The drawing under review shows one solid part. Ordinate dimensions are in mm from its lowest x, y, z. Coordinates: 2 decimals unless noted, no trailing zeros. Loops run counter-clockwise (first coordinate to the right, second up) from the corner with the lowest first, then second, coordinate; pieces in that order, holes last. Notation, with made-up numbers: M -2.75,83.25 L 35.25,83.25 A24 ccw 35.25,114.25 Z; hole C -23.5,1.25 d6. An arc over 180 degrees is marked long. Return JSON: item names as keys, results as strings.
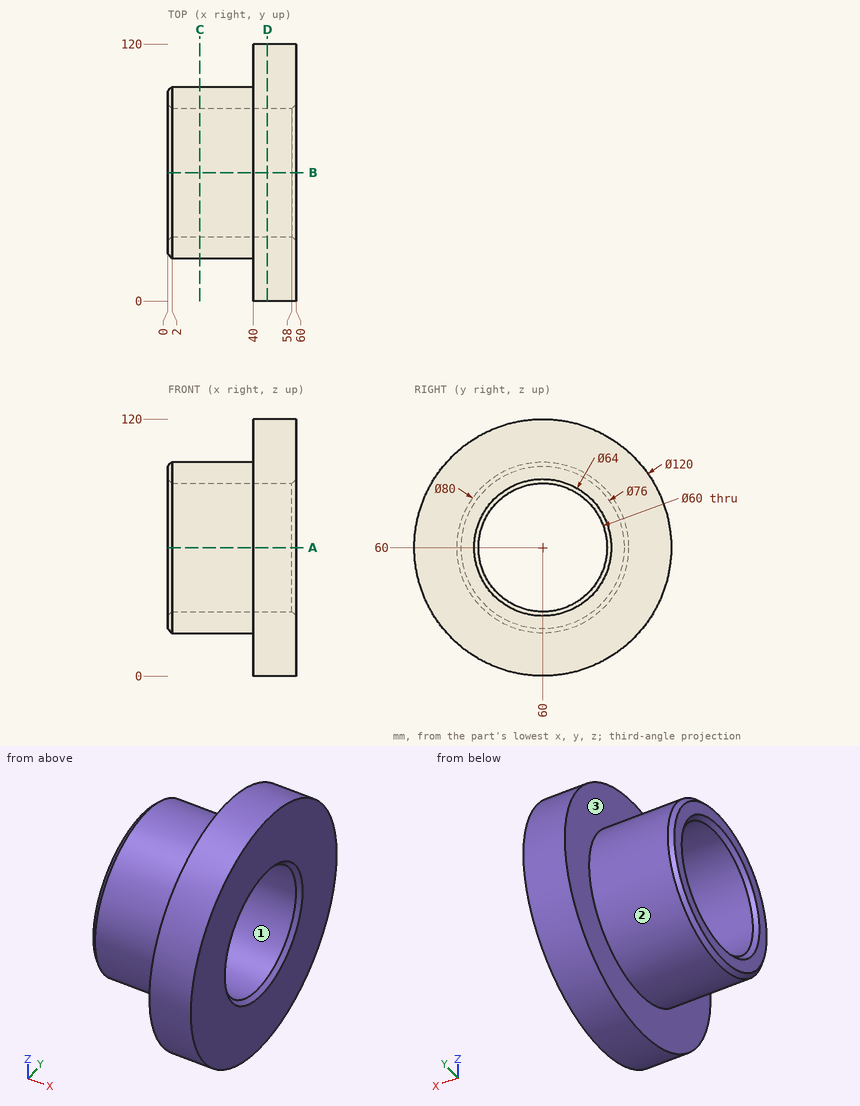
1. To check wall thickness, follow line 1 (Y direction, x = 28, z = 60); line 2 (X direction, y = 13, z = 48.5). State the ranges of each line that lie inside material, in increasing order.
Check values:
{"line 1": "20 to 30, 90 to 100", "line 2": "40 to 60"}
2. Insertion check: pin 1 Ø4 at (x, y) = (54, 80.5) entering from -Z; pin 2 Ø4 at (x, z) = (45, 65.5) entering from -Y; pin 3 Ø8 at (x, y) = (17.5, 78.5) entering from -Z. Each pin has a flat end and moves straight along its axis. Give the tip position at first contact, or say it passes through.
Check values:
{"pin 1": "z = 2.92", "pin 2": "y = 0.1", "pin 3": "z = 22.72"}
3. Add section C-C on x = 15. Give the boundary of the cut face in (y, z).
Check values:
{"outline": "C 60,60 d80; hole C 60,60 d60"}
4. Add section A-A on z = 60. Give the boundary of the cut face in (x, y).
Check values:
{"outline": "M 0,22 L 2,20 L 40,20 L 40,0 L 60,0 L 60,28 L 58,30 L 2,30 L 0,28 Z; M 0,92 L 2,90 L 58,90 L 60,92 L 60,120 L 40,120 L 40,100 L 2,100 L 0,98 Z"}
5. The part is to be moulded in two halves that separate along Y. For the marked faces 1, 2 and 3, say which applies: released by +Y, released by -Y, zero draft, split by the parting line, or undercut.
Check values:
{"face 1": "undercut", "face 2": "split by the parting line", "face 3": "zero draft"}
6. Add section D-D on x = 46.5. Give the boundary of the cut face in (y, z).
Check values:
{"outline": "C 60,60 d120; hole C 60,60 d60"}
